Can you work these out from the drawing? Everything is in mm from the part's minimum corner. A direction names the side the tool comes from. Give positions to 0.01 mm unless a question says otherwise; leave off trailing zeros. Write each loop counter-clockwise with the first axis right and the second up, starting at its lowest first coordinate (ties: lowest second). Pieces come first, ordered by that corner, then holes. Notation, with made-up numbers: (38, 51) -> (43, 51) arc R24 cw to (43, 83) -> close; hole circle Ø3 at (66, 80). An arc over 180 degrees is marked (long way). Write item = value, one per line. Start each with the question number.
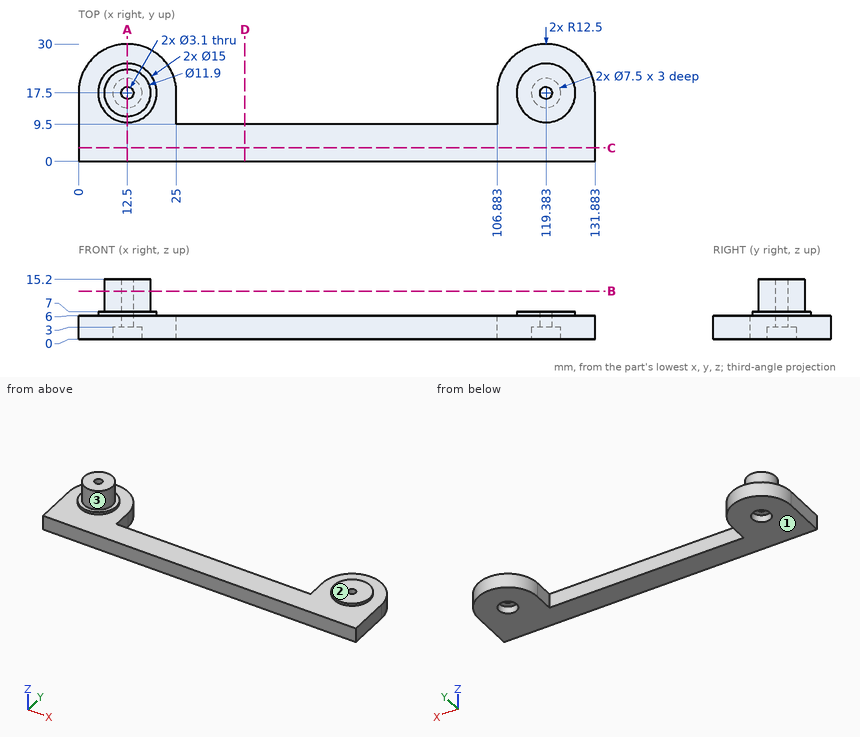
(1) Imagine slicing it at D-D (x = 42.5). Please give me the cut outline in (y, z), then the cut area to 3 significant figures.
(2) If I drill on line 1 along X through (y, z) = (13.5, 2.25); line 2 along X through (y, z) = (27.5, 4.75); line 3 along Y through (x, z) = (12.5, 1.6), over which ranges is the centre line in solid material (lowest first)? Write a range as from..to.
(3) Imagine slicing it at B-B (z = 12.25). Please give me the cut outline in (x, y), then the cut area to 3 significant figures.
(4) On a 3-axis mill with a long thin cutter (end or side, diameter ignored), from which of +Z, -Z, +X, -X, +Y, -Y can I reach the whole of each face in a straight line? I mean the marked faces 1, 2 and 3. Say none if no direction works.
(5) I'm going to push flat-ended pins straight in: pin 1 (6 mm diameter, centred on x = 91, y = 8.5, fed in from +Z); pin 2 (2 mm diameter, centred on x = 13.5, y = 18, fed in from -Z); pin 3 (10 mm diameter, centred on x = 119.38, y = 17.5, fed in from +Z). Where does each tip first touch, or does it pass through?
(6) Imagine slicing it at C-C (y = 3.5). Please give me the cut outline in (x, z).
(7) Imagine slicing it at A-A (x = 12.5). Please give me the cut outline in (y, z).
Answers below:
q1.outline = (0, 0) -> (9.5, 0) -> (9.5, 6) -> (0, 6) -> close
q1.area = 57.0 mm^2
q2.line_1 = 0..25, 106.88..131.88
q2.line_2 = 5..20, 111.88..126.88
q2.line_3 = 0..13.75, 21.25..30
q3.outline = circle Ø11.9 at (12.5, 17.5); hole circle Ø3.1 at (12.5, 17.5)
q3.area = 104 mm^2
q4.face_1 = -Z, +X, -X, +Y, -Y
q4.face_2 = +Z, +X, +Y, -Y
q4.face_3 = +Z
q5.pin_1 = 6
q5.pin_2 = 3
q5.pin_3 = 7
q6.outline = (0, 0) -> (131.88, 0) -> (131.88, 6) -> (0, 6) -> close
q7.outline = (0, 0) -> (13.75, 0) -> (13.75, 3) -> (15.95, 3) -> (15.95, 15.2) -> (11.55, 15.2) -> (11.55, 7) -> (10, 7) -> (10, 6) -> (0, 6) -> close; (19.05, 3) -> (21.25, 3) -> (21.25, 0) -> (30, 0) -> (30, 6) -> (25, 6) -> (25, 7) -> (23.45, 7) -> (23.45, 15.2) -> (19.05, 15.2) -> close
